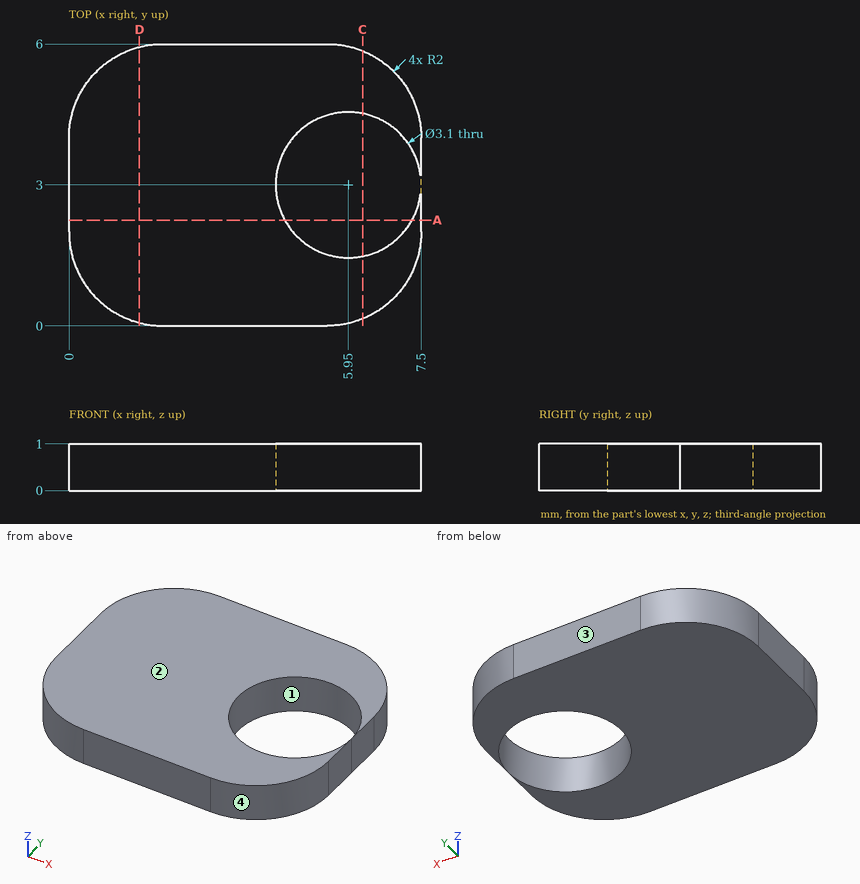
Drawing for the job (mm, zero at the part's lowest x, y, z). Coordinates: 2 decimals unless noted, no trailing zeros. Loops run counter-clockwise (first coordinate to the right, second up) from the corner with the lowest first, then second, coordinate; pieces in that order, holes last. Notation, with made-up numbers: (56.5, 10.25) - (103.5, 10.25) arc R14 ccw to (103.5, 14.25) - close; hole circle Ø9 at (51.5, 19.5). An arc over 180 degrees is marked (long way). Return JSON: item names as keys, results as strings.
1. Band-saw the part on D-D (x = 1.5). Give the cut face in (y, z).
Result:
{"outline": "(0.06, 0) - (5.94, 0) - (5.94, 1) - (0.06, 1) - close"}
2. Band-saw the part on A-A (y = 2.25). Give the cut face in (x, z).
Result:
{"outline": "(0, 0) - (4.59, 0) - (4.59, 1) - (0, 1) - close; (7.31, 0) - (7.5, 0) - (7.5, 1) - (7.31, 1) - close"}
3. Band-saw the part on C-C (x = 6.25). Give the cut face in (y, z), and give its area (3 significant figures).
Result:
{"outline": "(0.15, 0) - (1.48, 0) - (1.48, 1) - (0.15, 1) - close; (4.52, 0) - (5.85, 0) - (5.85, 1) - (4.52, 1) - close", "area": "2.67 mm2"}
4. Probe L1, parallel to Y at x = 5.95, z = 0.5; L2, parallel to X at y = 2, z = 0.7; L3, parallel to Y at x = 6.75, z = 0.75. List the from-to ranges inside material, lowest first. Write a range as from..to.
Result:
{"L1": "y = 0.05..1.45, 4.55..5.95", "L2": "x = 0..4.77, 7.13..7.5", "L3": "y = 0.44..1.67, 4.33..5.56"}
5. Drop flat-ended pins along their axis: pin 1 (3 mm diameter, centred on x = 6.5, y = 3.5, fed in from +Z); pin 2 (1.9 mm diameter, centred on x = 5.95, y = 3, fed in from -Z). Give the stop position or say it passes through.
Result:
{"pin 1": "stops at z = 1", "pin 2": "passes through"}
6. Mould opens along Y. For the marked faces 1, 2, 3 and 4 say: released by +Y, released by -Y, zero draft, split by the parting line, or undercut.
Result:
{"face 1": "undercut", "face 2": "zero draft", "face 3": "released by +Y", "face 4": "released by -Y"}
